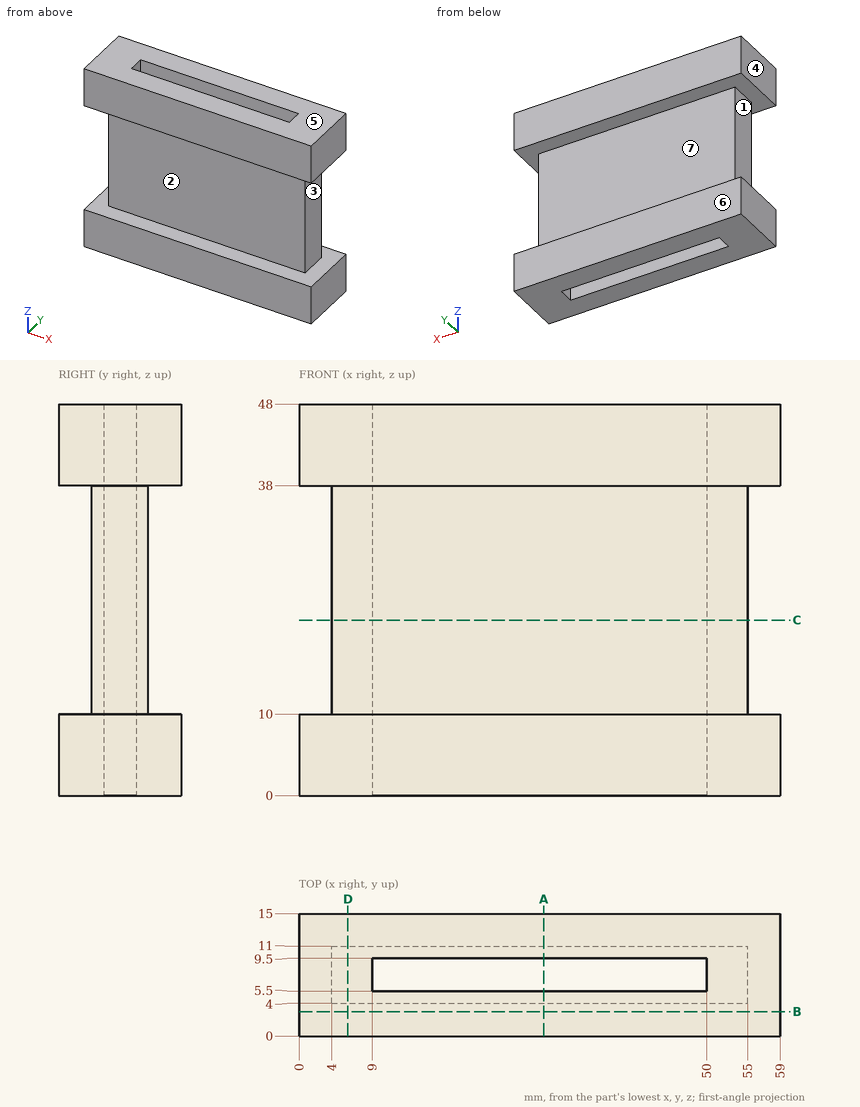
Answer from the drawing. Dimensions are ordinates in mm from the lowest x, y and z of the part. A direction names the side the tool comes from. Give positions to 0.01 mm unless a question says otherwise; leave off trailing zeros. Order: outer loops, then holes, each group sorted by start corner. A loop starts at its lowest first (then second) coordinate and runs counter-clockwise, first axis right, second up. Notation, with made-up numbers: (29, 17) - (64, 17) arc R11 cw to (64, 26) - close; hole circle Ø3 at (-23, 79). An arc over 180 degrees is marked (long way). One line per item, written item: value. Start each with the question number.
1. Which of the six approach directions +Z, -Z, +X, -X, +Y, -Y give full straight-line access (tool end or side, diameter ignored) to the marked faces 1, 2, 3 and 4?
2. Each of these flat-tipped pins is pushed along its axis until it touches: pin 1 Ø7.5 at (y, z) = (6, 20) entering from +X; pin 2 Ø4 at (x, y) = (15.5, 5.5) entering from -Z; pin 3 Ø10 at (x, z) = (52, 16) entering from +Y; pin 4 Ø3.5 at (y, z) = (7.5, 20) entering from -X. Where does it stop, or does it pass through?
3. Section D-D, the plane x = 6 is taken. Write down the section's boundary in (y, z).
4. Consider line 1 (Y direction, x = 30.5, z = 27.5); line 2 (X direction, y = 7, z = 5.5); line 3 (Y direction, x = 27.5, z = 7). Determine where each line is inside the solid, lowest interval first.
5. Section A-A, the plane x = 30 is taken. Write down the section's boundary in (y, z).
6. Section C-C, the plane z = 21.5 is taken. Write down the section's boundary in (x, y), then the cut area to 3 significant figures.
7. Section B-B, the plane y = 3 is taken. Write down the section's boundary in (x, z), then the cut area to 3 significant figures.
8. For a pull along Z with two mould halves and no side action, classify the marked faces 5, 6 and 7 as released by +Z, released by -Z, zero draft, split by the parting line, or undercut.
Filled sheet:
1. face 1: -X, +Y, -Y
1. face 2: +X, -X, -Y
1. face 3: +X, +Y, -Y
1. face 4: +Z, -Z, -X, +Y, -Y
2. pin 1: x = 55
2. pin 2: z = 0
2. pin 3: y = 11
2. pin 4: x = 4
3. outline: (0, 0) - (15, 0) - (15, 10) - (11, 10) - (11, 38) - (15, 38) - (15, 48) - (0, 48) - (0, 38) - (4, 38) - (4, 10) - (0, 10) - close
4. line 1: 4 to 5.5, 9.5 to 11
4. line 2: 0 to 9, 50 to 59
4. line 3: 0 to 5.5, 9.5 to 15
5. outline: (0, 0) - (5.5, 0) - (5.5, 48) - (0, 48) - (0, 38) - (4, 38) - (4, 10) - (0, 10) - close; (9.5, 0) - (15, 0) - (15, 10) - (11, 10) - (11, 38) - (15, 38) - (15, 48) - (9.5, 48) - close
6. outline: (4, 4) - (55, 4) - (55, 11) - (4, 11) - close; hole (9, 5.5) - (50, 5.5) - (50, 9.5) - (9, 9.5) - close
6. area: 193 mm²
7. outline: (0, 0) - (59, 0) - (59, 10) - (0, 10) - close; (0, 38) - (59, 38) - (59, 48) - (0, 48) - close
7. area: 1,180 mm²
8. face 5: released by +Z
8. face 6: zero draft
8. face 7: undercut
